Build history of the part. All positions in model axes, mm. Give positions to 0.01 mm unless a question says otherwise; leave off trailing zeros. Loops run counter-clockwise (first coordinate to the right, second up) from the corner with the lowest first, then second, coordinate; pieces in that order, holes last. Notation, with made-up numbers: (-38.5, -26) - (-31.5, -26) arc R6 cw to (-31.5, -21) - close; hole circle Ø8 at (60, -31.5). An arc over 180 degrees is marked (long way). Return JSON: item names as keys, results as strings. Group by question number.
1) Drop flat-ended pins along their axis: pin 1 (0.5 mm diameter, centred on y = 0.5, z = -52, fed in from +X); pin 2 (5.5 mm diameter, centred on x = 212.5, z = 74, fed in from -Y). Give the stop position or say it passes through.
2) Slice it at A-A (z = 101.5). List the corners of the cut face in (x, y), and give its area (3 significant figures).
3) Slice it at B-B (y = 0.3). List the corners of the cut face in (x, z).
4) Drill centre line: probe 1 along X at (y, z) = (0.3, 129.5). Where is it in solid material? Low to high. Write a range as from..to.
```python
from build123d import *

# Parameters (mm, degrees)
SKETCH1_W           = 430
SKETCH1_H           = 310
BOSS_EXTRUDE1_DEPTH = 2
SKETCH2_W           = 7
SKETCH2_H           = 1
CUT_EXTRUDE1_DEPTH  = 311


with BuildPart() as part:
    # Sketch1 → Boss-Extrude1 (new body)
    with BuildSketch(Plane(origin=(0, 0, 0), x_dir=(1, 0, 0), z_dir=(0, 1, 0))):
        Rectangle(SKETCH1_W, SKETCH1_H)
    extrude(amount=BOSS_EXTRUDE1_DEPTH)

    # Sketch2 → Cut-Extrude1 (cut, through all)
    with BuildSketch(Plane.XY.offset(155)):
        with Locations((-211.5, 0.5)):
            Rectangle(SKETCH2_W, SKETCH2_H)
        with Locations((211.5, 0.5)):
            Rectangle(SKETCH2_W, SKETCH2_H)
    extrude(amount=-CUT_EXTRUDE1_DEPTH, mode=Mode.SUBTRACT)


solid = part.part
```
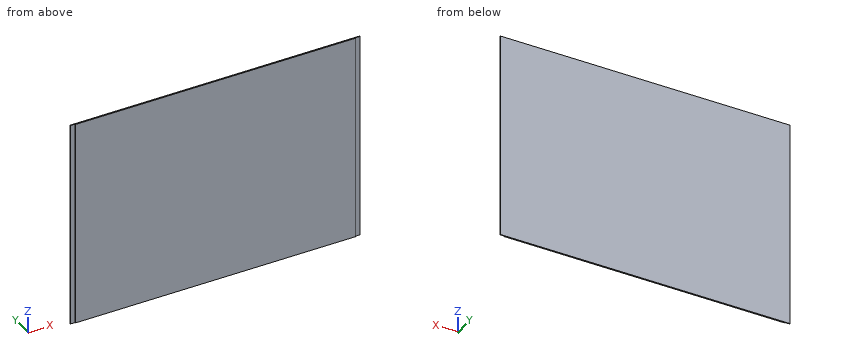
Results:
{
 "1": {"pin 1": "x = 208", "pin 2": "y = 1"},
 "2": {"outline": "(-215, 1) - (-208, 1) - (-208, 0) - (208, 0) - (208, 1) - (215, 1) - (215, 2) - (-215, 2) - close", "area": "846 mm2"},
 "3": {"outline": "(-208, -155) - (208, -155) - (208, 155) - (-208, 155) - close"},
 "4": {"probe 1": "-208..208"}
}
